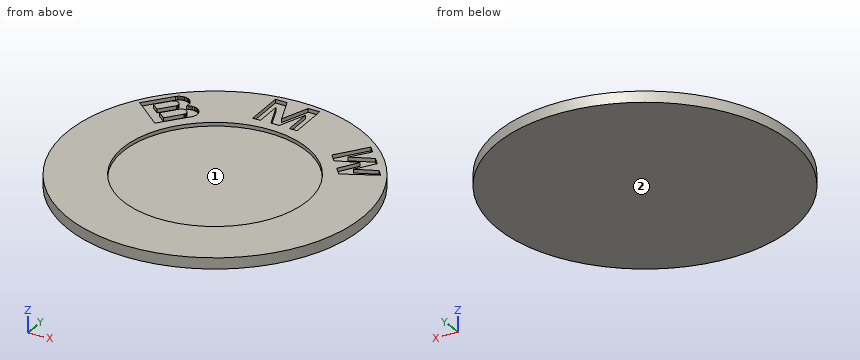
from build123d import *

# Parameters (mm, degrees)
SKETCH_1_R          = 40.2
EXTRUDE_1_DEPTH     = 3
CUT_EXTRUDE_2_DEPTH = 1
CUT_EXTRUDE_START   = -3
SKETCH_2_R          = 25.115
CUT_EXTRUDE_1_DEPTH = 1


with BuildPart() as part:
    # 草图1 → 凸台-拉伸1 (new body)
    with BuildSketch(Plane.XY):
        Circle(SKETCH_1_R)
    extrude(amount=EXTRUDE_1_DEPTH)

    # 草图4 → 切除-拉伸2 (cut)
    # profile 1 of 3: a face of its own
    with BuildSketch(Plane.XY.offset(3)):
        Polygon((-32.5857633, 21.06745862), (-24.581820031, 14.318573463), (-18.667207086, 21.333098879), (-18.41413244, 21.736159792), (-18.234803522, 22.177001467), (-18.13465246, 22.642257204), (-18.116731012, 23.117843142), (-18.181557978, 23.589339724), (-18.32718786, 24.042434206), (-18.549203241, 24.463393679), (-18.840867365, 24.839477053), (-19.193337763, 25.159270754), (-19.595940912, 25.413070192), (-20.036454523, 25.593200197), (-20.501542414, 25.694198122), (-20.977090204, 25.712981691), (-21.448693598, 25.649001589), (-21.902055109, 25.504195681), (-22.323418939, 25.282943239), (-22.237939203, 25.721435061), (-22.226228083, 26.168029299), (-22.288621271, 26.610396853), (-22.423394525, 27.03633069), (-22.626817072, 27.434081545), (-22.893288935, 27.792647829), (-23.215455377, 28.102157106), (-23.584405268, 28.354064455), (-23.989976251, 28.541396608), (-24.420968378, 28.659011354), (-24.865479792, 28.703643312), (-25.311242426, 28.67405652), (-25.745965326, 28.571090212), (-26.157632196, 28.397567263), (-26.534890497, 28.158278933), (-26.867333734, 27.859832277), align=None)
        Polygon((-29.433129633, 22.00672864), (-27.536842846, 20.401686478), (-24.415383661, 24.089553347), (-24.332948053, 24.288070192), (-24.284310663, 24.497451296), (-24.270799005, 24.71198987), (-24.292779291, 24.925811281), (-24.349656427, 25.133101931), (-24.439881647, 25.328216066), (-24.560983026, 25.505813112), (-24.709672296, 25.661040773), (-24.88187536, 25.789687624), (-25.07290777, 25.888244143), (-25.277558649, 25.953994265), (-25.490235651, 25.985183229), (-25.705155695, 25.980926027), (-25.916436518, 25.941359987), (-26.118325556, 25.867568483), (-26.305306757, 25.761535158), (-26.472298944, 25.626189699), (-26.614724481, 25.465194216), (-26.728715265, 25.282943239), align=None, mode=Mode.SUBTRACT)
        Polygon((-22.927964533, 23.086165895), (-26.131158197, 19.230041018), (-24.13251623, 17.548820009), (-20.844605768, 21.457534304), (-20.737939203, 21.661635866), (-20.668130243, 21.881103029), (-20.637284601, 22.109313479), (-20.646325434, 22.339431276), (-20.694978083, 22.564528933), (-20.781777704, 22.777846804), (-20.904122675, 22.972960939), (-21.058335626, 23.143996706), (-21.239770258, 23.285842409), (-21.442979181, 23.39419507), (-21.661851251, 23.465835085), (-21.889809931, 23.498580446), (-22.119996393, 23.491454592), (-22.345490778, 23.444686403), (-22.559518183, 23.359664431), (-22.755639398, 23.23895215), align=None, mode=Mode.SUBTRACT)
    # profile 2 of 3: a face of its own
    with BuildSketch(Plane.XY.offset(3)):
        Polygon((-5.996850336, 38.408904543), (-5.996850336, 27.859832277), (-3.91276153, 27.859832277), (-3.91276153, 35.218716958), (-1.150554499, 27.972180703), (1.12643067, 27.972180703), (3.939782293, 35.218721034), (3.939782293, 27.859832277), (6.014273321, 27.859832277), (6.014273321, 38.408905525), (2.876387274, 38.408905525), (0, 31), (-2.824097956, 38.408904543), align=None)
    # profile 3 of 3: a face of its own
    with BuildSketch(Plane.XY.offset(3)):
        Polygon((24.872824347, 29.687392702), (26.402881435, 27.859829995), (22.690074891, 22.851733117), (28.558242873, 25.479165769), (30.175307816, 23.547677324), (26.718580446, 18.404779635), (32.2027141, 20.860263506), (33.683638635, 19.091386728), (24.872830811, 14.723630109), (23.099783575, 16.841430178), (26.402884161, 22.00672864), (20.684073126, 19.667968264), (18.909277594, 21.787856569), align=None)
    extrude(amount=-CUT_EXTRUDE_2_DEPTH, mode=Mode.SUBTRACT)

    # 草图2 → 切除-拉伸1 (cut)
    with BuildSketch(Plane(origin=(0, 0, 0), x_dir=(-1, 0, 0), z_dir=(0, 0, -1)).offset(CUT_EXTRUDE_START)):
        with Locations(Location((0, 0, 0), (0, 0, 180))):
            Circle(SKETCH_2_R)
    extrude(amount=CUT_EXTRUDE_1_DEPTH, mode=Mode.SUBTRACT)


solid = part.part
Model file for the job. Use its own axes, mm. Face numbers are marked on the shaded views. Round coordinates to 2 decimals unless told otherwise and drop trailing zeros. Loops run counter-clockwise (first coordinate to the right, second up) from the corner with the lowest first, then second, coordinate; pieces in that order, holes last. Notation, with made-up numbers: (62, -13) -> (120, -13) arc R13 cw to (120, -3) -> close; hole circle Ø5 at (-21, -19). An arc over 180 degrees is marked (long way). Answer as CSV lines item,"result". Start each with the question number.
1) Slice it at B-B (y = 0). List the corners of the cut face in (x, z) (3 decimals), plus the area to 3 significant figures.
2) Probe line 1 along Z through (x, y) = (-20.5, 19.5); line 2 along Y through (x, z) = (-4, 2.2); line 3 along X through (y, z) = (-12, 2.65). List the from-to ranges inside material, lowest first.
3) Slice it at C-C (x = -16). List the corners of the cut face in (y, z), plus the area to 3 significant figures.
4) Pin check, flat tips, straight feed: P1, Ø0.8, axis at y = 30.5, z = 2.5, coming from the +X side; P2, Ø0.5, axis at x = -5.5, z = 2.5, coming from the +Y side; P3, Ø0.5, axis at y = 32, z = 2.5, coming from the -X side. Stop position of each tip, or through.
5) Mould opens along Y. For the marked faces 1 and 2 say: +Y half, -Y half, draft (parallel to the pull), parting line (faces both ways), or undercut.
6) Slice it at D-D (y = 34). List the corners of the cut face in (x, z).
7) Slice it at A-A (z = 2.45). State how many separate pieces and enclosed holes the cut face has, plus the area to 3 significant figures.
Filled in:
1,outline,"(-40.2, 0) -> (40.2, 0) -> (40.2, 3) -> (25.115, 3) -> (25.115, 2) -> (-25.115, 2) -> (-25.115, 3) -> (-40.2, 3) -> close"
1,area,"191 mm2"
2,line 1,"z = 0 to 2"
2,line 2,"y = -40 to -24.79, 24.79 to 27.86, 38.41 to 40"
2,line 3,"x = -38.37 to -22.06, 22.06 to 38.37"
3,outline,"(-36.88, 0) -> (36.88, 0) -> (36.88, 3) -> (19.36, 3) -> (19.36, 2) -> (-19.36, 2) -> (-19.36, 3) -> (-36.88, 3) -> close"
3,area,"183 mm2"
4,P1,"stops at x = 26.65"
4,P2,"stops at y = 39.86"
4,P3,"stops at x = -24.66"
5,face 1,"undercut"
5,face 2,"draft"
6,outline,"(-21.45, 0) -> (21.45, 0) -> (21.45, 3) -> (6.01, 3) -> (6.01, 2) -> (3.94, 2) -> (3.94, 3) -> (3.47, 3) -> (3.47, 2) -> (1.16, 2) -> (1.16, 3) -> (-1.14, 3) -> (-1.14, 2) -> (-3.45, 2) -> (-3.45, 3) -> (-3.91, 3) -> (-3.91, 2) -> (-6, 2) -> (-6, 3) -> (-21.45, 3) -> close"
7,separate pieces,"3"
7,enclosed holes,"4"
7,area,"2,840 mm2"
